Geometry check sheet. Reference: the model listing, model coordinates, mm. Face numbers are marked on the shaded views. A direction names the side the tool comes from. Round coordinates to 2 decimals unless told otherwise and drop trailing zeros. Loops run counter-clockwise (first coordinate to the right, second up) from the corner with the lowest first, then second, coordinate; pieces in that order, holes last.
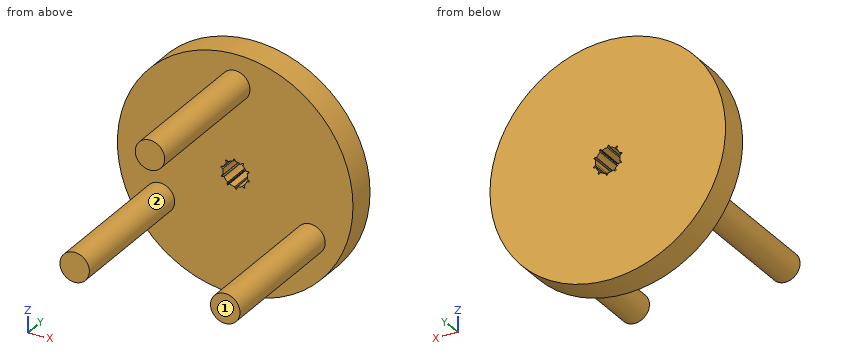
```python
from build123d import *

# Parameters (mm, degrees)
F0_R     = 20
F1_DEPTH = 5
F2_R     = 2.5
F3_DEPTH = 25


with BuildPart() as f1:
    # F0 (on Front) → F1 (new body)
    with BuildSketch(Plane.XZ):
        Circle(F0_R)
        with BuildLine():
            ThreePointArc((2.022994, 0.617024), (2.091872, 0.311923), (2.115, 0))
            ThreePointArc((2.115, 0), (2.107794, -0.17444), (2.086225, -0.347692))
            ThreePointArc((2.086225, -0.347692), (2.181907, -0.376409), (2.271319, -0.420964))
            ThreePointArc((2.271319, -0.420964), (2.360037, -0.487855), (2.433965, -0.570799))
            Line((2.433965, -0.570799), (2.411372, -0.65976))
            ThreePointArc((2.411372, -0.65976), (2.306825, -0.697377), (2.196941, -0.713829))
            ThreePointArc((2.196941, -0.713829), (2.097104, -0.710321), (1.999314, -0.689903))
            ThreePointArc((1.999314, -0.689903), (1.788714, -1.128595), (1.483424, -1.507541))
            ThreePointArc((1.483424, -1.507541), (1.543952, -1.587014), (1.590099, -1.675615))
            ThreePointArc((1.590099, -1.675615), (1.622556, -1.781878), (1.633612, -1.892435))
            Line((1.633612, -1.892435), (1.563044, -1.951126))
            ThreePointArc((1.563044, -1.951126), (1.456352, -1.920108), (1.357784, -1.868829))
            ThreePointArc((1.357784, -1.868829), (1.279077, -1.807308), (1.211964, -1.733311))
            ThreePointArc((1.211964, -1.733311), (0.783729, -1.964432), (0.314005, -2.091561))
            ThreePointArc((0.314005, -2.091561), (0.31626, -2.191433), (0.301516, -2.290238))
            ThreePointArc((0.301516, -2.290238), (0.265314, -2.395284), (0.209274, -2.491225))
            Line((0.209274, -2.491225), (0.117686, -2.497228))
            ThreePointArc((0.117686, -2.497228), (0.049603, -2.409422), (0, -2.31))
            ThreePointArc((0, -2.31), (-0.027515, -2.213966), (-0.038315, -2.114653))
            ThreePointArc((-0.038315, -2.114653), (-0.520614, -2.049923), (-0.975353, -1.876675))
            ThreePointArc((-0.975353, -1.876675), (-1.032233, -1.9588), (-1.102237, -2.030068))
            ThreePointArc((-1.102237, -2.030068), (-1.193269, -2.093773), (-1.294999, -2.138452))
            Line((-1.294999, -2.138452), (-1.372624, -2.089475))
            ThreePointArc((-1.372624, -2.089475), (-1.376094, -1.97842), (-1.357784, -1.868829))
            ThreePointArc((-1.357784, -1.868829), (-1.323596, -1.774963), (-1.273959, -1.688269))
            ThreePointArc((-1.273959, -1.688269), (-1.6261, -1.352413), (-1.89216, -0.944964))
            ThreePointArc((-1.89216, -0.944964), (-1.986447, -0.977971), (-2.084972, -0.994481))
            ThreePointArc((-2.084972, -0.994481), (-2.196064, -0.992512), (-2.304627, -0.968863))
            Line((-2.304627, -0.968863), (-2.338638, -0.883612))
            ThreePointArc((-2.338638, -0.883612), (-2.276169, -0.791728), (-2.196941, -0.713829))
            ThreePointArc((-2.196941, -0.713829), (-2.114109, -0.657985), (-2.022994, -0.617024))
            ThreePointArc((-2.022994, -0.617024), (-2.110472, -0.138328), (-2.086225, 0.347692))
            ThreePointArc((-2.086225, 0.347692), (-2.181907, 0.376409), (-2.271319, 0.420964))
            ThreePointArc((-2.271319, 0.420964), (-2.360037, 0.487855), (-2.433965, 0.570799))
            Line((-2.433965, 0.570799), (-2.411372, 0.65976))
            ThreePointArc((-2.411372, 0.65976), (-2.306825, 0.697377), (-2.196941, 0.713829))
            ThreePointArc((-2.196941, 0.713829), (-2.097104, 0.710321), (-1.999314, 0.689903))
            ThreePointArc((-1.999314, 0.689903), (-1.788714, 1.128595), (-1.483424, 1.507541))
            ThreePointArc((-1.483424, 1.507541), (-1.543952, 1.587014), (-1.590099, 1.675615))
            ThreePointArc((-1.590099, 1.675615), (-1.622556, 1.781878), (-1.633612, 1.892435))
            Line((-1.633612, 1.892435), (-1.563044, 1.951126))
            ThreePointArc((-1.563044, 1.951126), (-1.456352, 1.920108), (-1.357784, 1.868829))
            ThreePointArc((-1.357784, 1.868829), (-1.279077, 1.807308), (-1.211964, 1.733311))
            ThreePointArc((-1.211964, 1.733311), (-0.783729, 1.964432), (-0.314005, 2.091561))
            ThreePointArc((-0.314005, 2.091561), (-0.31626, 2.191433), (-0.301516, 2.290238))
            ThreePointArc((-0.301516, 2.290238), (-0.265314, 2.395284), (-0.209274, 2.491225))
            Line((-0.209274, 2.491225), (-0.117686, 2.497228))
            ThreePointArc((-0.117686, 2.497228), (-0.049603, 2.409422), (0, 2.31))
            ThreePointArc((0, 2.31), (0.027515, 2.213966), (0.038315, 2.114653))
            ThreePointArc((0.038315, 2.114653), (0.520614, 2.049923), (0.975353, 1.876675))
            ThreePointArc((0.975353, 1.876675), (1.032233, 1.9588), (1.102237, 2.030068))
            ThreePointArc((1.102237, 2.030068), (1.193269, 2.093773), (1.294999, 2.138452))
            Line((1.294999, 2.138452), (1.372624, 2.089475))
            ThreePointArc((1.372624, 2.089475), (1.376094, 1.97842), (1.357784, 1.868829))
            ThreePointArc((1.357784, 1.868829), (1.323596, 1.774963), (1.273959, 1.688269))
            ThreePointArc((1.273959, 1.688269), (1.6261, 1.352413), (1.89216, 0.944964))
            ThreePointArc((1.89216, 0.944964), (1.986447, 0.977971), (2.084972, 0.994481))
            ThreePointArc((2.084972, 0.994481), (2.196064, 0.992512), (2.304627, 0.968863))
            Line((2.304627, 0.968863), (2.338638, 0.883612))
            ThreePointArc((2.338638, 0.883612), (2.276169, 0.791728), (2.196941, 0.713829))
            ThreePointArc((2.196941, 0.713829), (2.114109, 0.657985), (2.022994, 0.617024))
        make_face(mode=Mode.SUBTRACT)
    extrude(amount=F1_DEPTH)

    # F2 (on face) → F3 (join)
    with BuildSketch(Plane.XZ.offset(5)):
        with Locations((0, 14.761444)):
            Circle(F2_R)
        with Locations((-12.783785, -7.380722)):
            Circle(F2_R)
        with Locations((12.783785, -7.380722)):
            Circle(F2_R)
    extrude(amount=F3_DEPTH)


solid = f1.part
```
1) Scan lines: line 1 along Y through (x, z) = (3, -13); line 2 along X through (y, z) = (-28.5, 17); line 3 along Z through (x, y) = (11.5, -6.25). Record each from-to range of solid material in increasing order.
Report:
line 1: y = -5 to 0
line 2: x = -1.11 to 1.11
line 3: z = -9.53 to -5.24
2) Gauge pin test, flat ends, axial feed: pin 1 (2 mm diameter, centred on x = -3, y = -23, fed in from +Z); pin 2 (5 mm diameter, centred on y = -21.5, z = -10.5, fed in from +X); pin 3 (2 mm diameter, centred on y = -5, z = 7.5, fed in from -X). Record the tip position at first contact, or that the pin passes through.
Report:
pin 1: stops at z = 16.26
pin 2: stops at x = 15.21
pin 3: stops at x = -18.91
3) Sectioned sample at D-D, the plane z = -12. Record the cut outline in (x, y), then the cut area to 3 significant figures.
Report:
outline: (-16, -5) - (16, -5) - (16, 0) - (-16, 0) - close
area: 160 mm2
4) Sectioned sample at C-C, the plane x = 17.5. Record the cut outline in (y, z), then the cut area to 3 significant figures.
Report:
outline: (-5, -9.68) - (0, -9.68) - (0, 9.68) - (-5, 9.68) - close
area: 96.8 mm2
5) Sectioned sample at A-A, the plane z = 16. Record the cut outline in (x, y), then the cut area to 3 significant figures.
Report:
outline: (-12, -5) - (-2.17, -5) - (-2.17, -30) - (2.17, -30) - (2.17, -5) - (12, -5) - (12, 0) - (-12, 0) - close
area: 229 mm2
6) Sectioned sample at B-B, the plane y = -9.75. Record the cut outline in (x, z), then the cut area to 3 significant figures.
Report:
outline: circle Ø5 at (-12.78, -7.38); circle Ø5 at (0, 14.76); circle Ø5 at (12.78, -7.38)
area: 58.9 mm2
7) Access from +Z, -Z, +X, -X, +Y, -Y to the whole of each face (thin tool, end or side, straight path). Record for the marked faces 1 and 2.
Report:
face 1: +Z, -Z, +X, -X, -Y
face 2: -Y
